Design review of the part shown in the three views and the two pictorial views. Dimensions are in mm from the part's minimum x, y and z. Give positions to 0.01 mm unless a question says otherwise; leave off trailing zeros. Order: outer loops, then holes, each group sorted by start corner. A loop starts at its lowest first (then second) coordinate and runs counter-clockwise, first axis right, second up. Notation, with made-up numbers: (3.25, 72.5) -> (45.25, 72.5) arc R3 cw to (45.25, 77.5) -> close; hole circle Ø10 at (-7, -23.5). An arc over 180 degrees is marked (long way). Use one line per item in the form item = value.
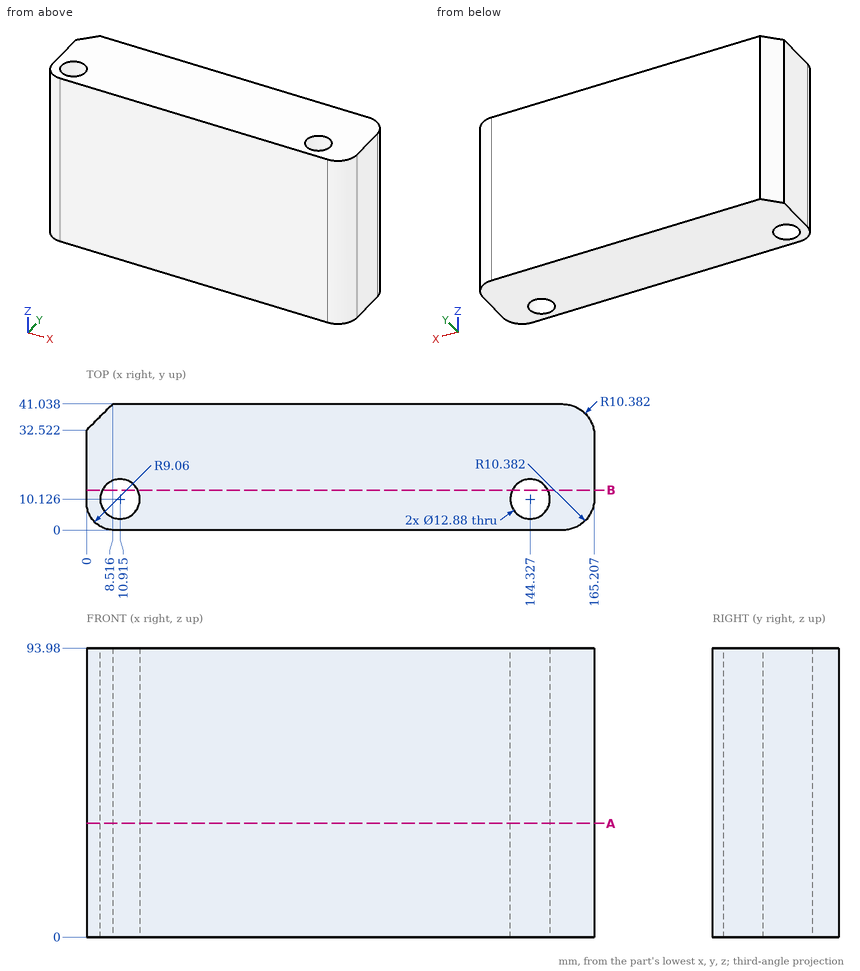
1. For L1, parallel to X at y = 7, z = 34.5 (1 decimal); L2, parallel to X at y = 5, z = 76 (1 decimal); L3, parallel to Y at x = 149, z = 26 (1 decimal), list the stretches that pass through material, from the lowest coordinate up.
Values:
L1 = 0.2 to 5.3, 16.5 to 138.7, 150 to 164.6
L2 = 1 to 7, 14.8 to 140.4, 148.2 to 163.7
L3 = 0 to 5.7, 14.6 to 41
2. Add section A-A on z = 37. Give the boundary of the cut face in (x, y) (1 decimal), then the cut area to 3 significant figures.
Values:
outline = (0, 9.1) arc R9.1 ccw to (9.1, 0) -> (154.8, 0) arc R10.4 ccw to (165.2, 10.4) -> (165.2, 30.7) arc R10.4 ccw to (154.8, 41) -> (8.5, 41) -> (0, 32.5) -> close; hole circle Ø12.9 at (10.9, 10.1); hole circle Ø12.9 at (144.3, 10.1)
area = 6,420 mm^2
3. Add section B-B on y = 13. Give the boundary of the cut face in (x, z).
Values:
outline = (0, 0) -> (5.15, 0) -> (5.15, 93.98) -> (0, 93.98) -> close; (16.68, 0) -> (138.56, 0) -> (138.56, 93.98) -> (16.68, 93.98) -> close; (150.09, 0) -> (165.21, 0) -> (165.21, 93.98) -> (150.09, 93.98) -> close
4. For pin 1 Ø3 at (y, z) = (6.5, 65) entering from -X, flat-tipped, find the tip position at first contact; note if it passes through.
Values:
pin_1 = 0.06
